Can you work these out from the model? Positions are in its coordinate system, mm. Face numbers are marked on the shaded views. A direction names the side the tool comes from. Give positions to 0.01 mm unless a question says otherwise; leave off trailing zeros. Loops run counter-clockwise (first coordinate to the right, second up) from the corner with the lowest first, then second, coordinate; pieces in that order, holes last. Notation, with made-up numbers: (87, -19.75) - (113, -19.75) arc R26 ccw to (113, 16.25) - close; hole circle Ø4 at (22.5, 37). An arc over 180 degrees is marked (long way). Answer as a JSON object with one key per item and string values.
```python
from build123d import *

# Parameters (mm, degrees)
SKETCH1_W           = 50
SKETCH1_H           = 50
SKETCH1_R           = 1.5
SKETCH1_R_2         = 1.646935024
SKETCH1_R_3         = 1.908192471
SKETCH1_R_4         = 1.759080553
EXTRUDE2_DEPTH      = 0.8
EXTRUDE3_DEPTH      = 10
EXTRUDE3_DEPTH_BACK = 7


with BuildPart() as part:
    # Sketch1 → Extrude2 (new, symmetric)
    with BuildSketch(Plane.XY):
        Rectangle(SKETCH1_W, SKETCH1_H)
        with Locations((-22, 22)):
            Circle(SKETCH1_R, mode=Mode.SUBTRACT)
        with Locations((22, 22)):
            Circle(SKETCH1_R_2, mode=Mode.SUBTRACT)
        with Locations((22, -22)):
            Circle(SKETCH1_R_3, mode=Mode.SUBTRACT)
        with Locations((-22, -22)):
            Circle(SKETCH1_R_4, mode=Mode.SUBTRACT)
    extrude(amount=EXTRUDE2_DEPTH, both=True)

    # Sketch2 → Extrude3 (add, two sides: drawn at the far end of the back side and taken through both)
    with BuildSketch(Plane.XY.offset(0.8).offset(-EXTRUDE3_DEPTH_BACK)):
        Polygon((-20, 20), (20, -20), (-20, -20), align=None)
        Polygon((-20, 20), (20, 20), (20, -20), align=None)
    extrude(amount=EXTRUDE3_DEPTH + EXTRUDE3_DEPTH_BACK)


solid = part.part
```
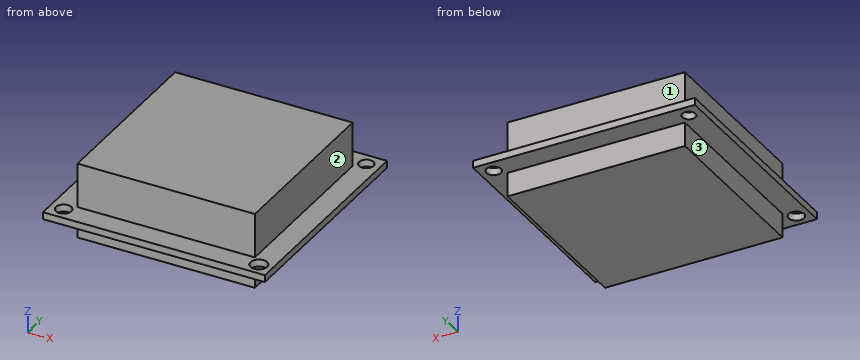
1) Imagine slicing it at A-A on x = -22. Write out the boundary of the cut face in (y, z), and give its area (3 significant figures).
Check sheet entries:
{"outline": "(-25, -0.8) - (-23.76, -0.8) - (-23.76, 0.8) - (-25, 0.8) - close; (-20.24, -0.8) - (20.5, -0.8) - (20.5, 0.8) - (-20.24, 0.8) - close; (23.5, -0.8) - (25, -0.8) - (25, 0.8) - (23.5, 0.8) - close", "area": "69.6 mm2"}
2) I'm going to push flat-ended pins straight in: P1, Ø5, axis at x = 13.5, z = 9, coming from the +Y side; P2, Ø4.5, axis at x = -22, y = -22, coming from the +Z side; P3, Ø4, axis at x = -11.5, z = -2, coming from the +Y side; P4, Ø3, axis at x = -7, z = 3.5, coming from the -Y side. Where does each tip first touch, or does it pass through?
Check sheet entries:
{"P1": "y = 20", "P2": "z = 0.8", "P3": "y = 25", "P4": "y = -20"}
3) Which directions (+Z, -Z, +X, -X, +Y, -Y) give clear straight access to the entire face, cutting with the end or side of a thin tool? Please do the marked faces 1, 2 and 3.
Check sheet entries:
{"face 1": "+Z, +X, -X, +Y", "face 2": "+Z, +X, +Y, -Y", "face 3": "-Z, -X, +Y, -Y"}
4) Imagine slicing it at B-B on y = -22. Write out the boundary of the cut face in (x, z).
Check sheet entries:
{"outline": "(-25, -0.8) - (-23.76, -0.8) - (-23.76, 0.8) - (-25, 0.8) - close; (-20.24, -0.8) - (20.09, -0.8) - (20.09, 0.8) - (-20.24, 0.8) - close; (23.91, -0.8) - (25, -0.8) - (25, 0.8) - (23.91, 0.8) - close"}
5) Imagine slicing it at C-C on x = 8. Write out the boundary of the cut face in (y, z).
Check sheet entries:
{"outline": "(-25, -0.8) - (-20, -0.8) - (-20, -6.2) - (20, -6.2) - (20, -0.8) - (25, -0.8) - (25, 0.8) - (20, 0.8) - (20, 10.8) - (-20, 10.8) - (-20, 0.8) - (-25, 0.8) - close"}
6) I need wall thicknesses on L1, parallel to Y at x = -22, z = 0.1; L2, parallel to Y at x = 22, z = 0; L3, parallel to X at y = -7, z = -2.25. Which ranges of each line are inside material? Lowest first, please.
Check sheet entries:
{"L1": "-25 to -23.76, -20.24 to 20.5, 23.5 to 25", "L2": "-25 to -23.91, -20.09 to 20.35, 23.65 to 25", "L3": "-20 to 20"}
